Can you work these out from the model? Positions are in its coordinate system, mm. Coordinates: 2 decimals unless noted, no trailing zeros. Loops run counter-clockwise (first coordinate to the right, second up) from the corner with the lowest first, then second, coordinate; pieces in that order, holes last.
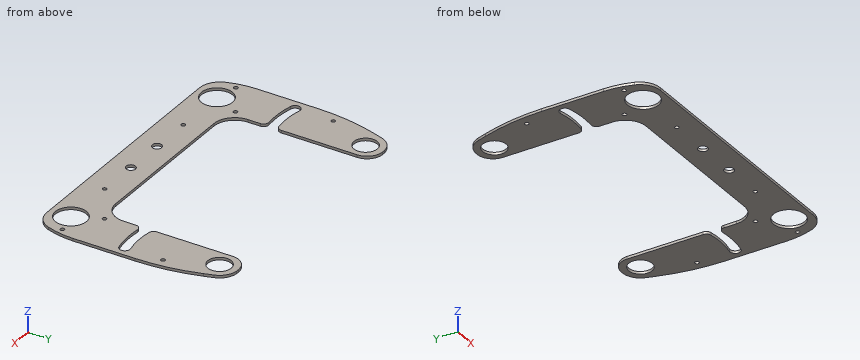
```python
from build123d import *

# Parameters (mm, degrees)
SKETCH1_R           = 14.2875
SKETCH1_R_2         = 19.05
SKETCH1_R_3         = 2.4892
SKETCH1_R_4         = 5.715
BOSS_EXTRUDE3_DEPTH = 3.175
SKETCH2_W           = 355.6
SKETCH2_H           = 19.05
CUT_EXTRUDE1_DEPTH  = 290.621961572
FILLET1_R           = 19.05
CUT_EXTRUDE2_DEPTH  = 290.621961572
FILLET2_R           = 254
CUT_EXTRUDE3_DEPTH  = 290.621961572
FILLET3_R           = 25.4
CUT_EXTRUDE4_DEPTH  = 290.621961572
FILLET4_R           = 6.35


with BuildPart() as part:
    # Sketch1 → Boss-Extrude3 (new body)
    with BuildSketch(Plane.XY):
        with BuildLine():
            Line((120.65, -152.4), (120.65, -6.35))
            Line((120.65, -6.35), (120.65, 6.35))
            ThreePointArc((120.65, 6.35), (124.369743879, 15.330256121), (133.35, 19.05))
            Line((133.35, 19.05), (165.1, 19.05))
            ThreePointArc((165.1, 19.05), (174.080256121, 15.330256121), (177.8, 6.35))
            Line((177.8, 6.35), (177.8, -6.35))
            Line((177.8, -6.35), (177.8, -222.25))
            ThreePointArc((177.8, -222.25), (175.940128061, -226.740128061), (171.45, -228.6))
            Line((171.45, -228.6), (12.7, -228.6))
            Line((12.7, -228.6), (-12.7, -228.6))
            Line((-12.7, -228.6), (-171.45, -228.6))
            ThreePointArc((-171.45, -228.6), (-175.940128061, -226.740128061), (-177.8, -222.25))
            Line((-177.8, -222.25), (-177.8, -6.35))
            Line((-177.8, -6.35), (-177.8, 6.35))
            ThreePointArc((-177.8, 6.35), (-174.080256121, 15.330256121), (-165.1, 19.05))
            Line((-165.1, 19.05), (-133.35, 19.05))
            ThreePointArc((-133.35, 19.05), (-124.369743879, 15.330256121), (-120.65, 6.35))
            Line((-120.65, 6.35), (-120.65, -6.35))
            Line((-120.65, -6.35), (-120.65, -152.4))
            ThreePointArc((-120.65, -152.4), (-113.210512242, -170.360512242), (-95.25, -177.8))
            Line((-95.25, -177.8), (-12.7, -177.8))
            Line((-12.7, -177.8), (12.7, -177.8))
            Line((12.7, -177.8), (95.25, -177.8))
            ThreePointArc((95.25, -177.8), (113.210512242, -170.360512242), (120.65, -152.4))
        make_face()
        with Locations((141.605, -22.02688)):
            Circle(SKETCH1_R, mode=Mode.SUBTRACT)
        with Locations(Location((-141.605, -22.02688, 0), (0, 0, 180))):
            Circle(SKETCH1_R, mode=Mode.SUBTRACT)
        with Locations((-141.605, -203.2)):
            Circle(SKETCH1_R_2, mode=Mode.SUBTRACT)
        with Locations(Location((141.605, -203.2, 0), (0, 0, 180))):
            Circle(SKETCH1_R_2, mode=Mode.SUBTRACT)
        with Locations((-76.2, -203.2)):
            Circle(SKETCH1_R_3, mode=Mode.SUBTRACT)
        with Locations(Location((76.2, -203.2, 0), (0, 0, 180))):
            Circle(SKETCH1_R_3, mode=Mode.SUBTRACT)
        with Locations((-25.4, -203.2)):
            Circle(SKETCH1_R_4, mode=Mode.SUBTRACT)
        with Locations((-149.225, 6.35)):
            Circle(SKETCH1_R_3, mode=Mode.SUBTRACT)
        with Locations(Location((149.225, 6.35, 0), (0, 0, 180))):
            Circle(SKETCH1_R_3, mode=Mode.SUBTRACT)
        with Locations((-168.275, -196.85)):
            Circle(SKETCH1_R_3, mode=Mode.SUBTRACT)
        with Locations(Location((168.275, -196.85, 0), (0, 0, 180))):
            Circle(SKETCH1_R_3, mode=Mode.SUBTRACT)
        with Locations((-165.1, -76.2)):
            Circle(SKETCH1_R_3, mode=Mode.SUBTRACT)
        with Locations(Location((165.1, -76.2, 0), (0, 0, 180))):
            Circle(SKETCH1_R_3, mode=Mode.SUBTRACT)
        with Locations((-127, -171.45)):
            Circle(SKETCH1_R_3, mode=Mode.SUBTRACT)
        with Locations(Location((127, -171.45, 0), (0, 0, 180))):
            Circle(SKETCH1_R_3, mode=Mode.SUBTRACT)
        with Locations(Location((25.4, -203.2, 0), (0, 0, 180))):
            Circle(SKETCH1_R_4, mode=Mode.SUBTRACT)
    extrude(amount=BOSS_EXTRUDE3_DEPTH)

    # Sketch2 → Cut-Extrude1 (cut, through all)
    with BuildSketch(Plane.XY.offset(3.175)):
        with Locations((0, 9.525)):
            Rectangle(SKETCH2_W, SKETCH2_H)
    extrude(amount=-CUT_EXTRUDE1_DEPTH, mode=Mode.SUBTRACT)

    # Fillet1
    fillet1_edges = [part.edges().sort_by_distance(p)[0] for p in [
        (-177.8, 0, 1.5875),
        (120.65, 0, 1.5875),
        (177.8, 0, 1.5875),
        (-120.65, 0, 1.5875),
    ]]
    fillet(fillet1_edges, radius=FILLET1_R)

    # Sketch3 → Cut-Extrude2 (cut, through all)
    with BuildSketch(Plane.XY.offset(3.175)):
        with BuildLine():
            Line((-177.8, 0), (-177.8, -63.5))
            Line((-177.8, -63.5), (-162.698792053, -15.403859213))
            ThreePointArc((-162.698792053, -15.403859213), (-155.445369527, -4.785747819), (-143.51, 0))
            Line((-143.51, 0), (-177.8, 0))
        make_face()
    cut_extrude2 = extrude(amount=-CUT_EXTRUDE2_DEPTH, mode=Mode.SUBTRACT)

    # Mirror1: Cut-Extrude2 across plane
    add(cut_extrude2.mirror(Plane.ZY), mode=Mode.SUBTRACT)

    # Fillet2
    fillet2_edges = [part.edges().sort_by_distance(p)[0] for p in [
        (-177.8, -63.5, 1.5875),
        (177.8, -63.5, 1.5875),
    ]]
    fillet(fillet2_edges, radius=FILLET2_R)

    # Sketch4 → Cut-Extrude3 (cut, through all)
    with BuildSketch(Plane.XY.offset(3.175)):
        with BuildLine():
            Line((-177.8, -177.8), (-177.8, -228.6))
            Line((-177.8, -228.6), (-164.188181024, -228.6))
            ThreePointArc((-164.188181024, -228.6), (-174.338063951, -204.096014982), (-177.8, -177.8))
        make_face()
        with BuildLine():
            Line((177.8, -177.8), (177.8, -228.6))
            Line((177.8, -228.6), (164.188181024, -228.6))
            ThreePointArc((164.188181024, -228.6), (174.338063951, -204.096014982), (177.8, -177.8))
        make_face()
    extrude(amount=-CUT_EXTRUDE3_DEPTH, mode=Mode.SUBTRACT)

    # Fillet3
    fillet3_edges = [part.edges().sort_by_distance(p)[0] for p in [
        (-164.188181024, -228.6, 1.5875),
        (164.188181024, -228.6, 1.5875),
    ]]
    fillet(fillet3_edges, radius=FILLET3_R)

    # Sketch5 → Cut-Extrude4 (cut, through all)
    with BuildSketch(Plane.XY.offset(3.175)):
        with BuildLine():
            Line((-120.65, -129.796193121), (-120.65, -116.826181287))
            ThreePointArc((-120.65, -116.826181287), (-142.167804376, -119.112938735), (-163.657650988, -116.576867488))
            ThreePointArc((-163.657650988, -116.576867488), (-171.284022099, -121.318540575), (-166.542349012, -128.944911687))
            ThreePointArc((-166.542349012, -128.944911687), (-143.641159604, -131.795686724), (-120.65, -129.796193121))
        make_face()
        with BuildLine():
            Line((120.65, -129.796193121), (120.65, -116.826181287))
            ThreePointArc((120.65, -116.826181287), (142.167804376, -119.112938735), (163.657650988, -116.576867488))
            ThreePointArc((163.657650988, -116.576867488), (171.284022099, -121.318540575), (166.542349012, -128.944911687))
            ThreePointArc((166.542349012, -128.944911687), (143.641159604, -131.795686724), (120.65, -129.796193121))
        make_face()
    extrude(amount=-CUT_EXTRUDE4_DEPTH, mode=Mode.SUBTRACT)

    # Fillet4
    fillet4_edges = [part.edges().sort_by_distance(p)[0] for p in [
        (-120.65, -116.826181287, 1.5875),
        (-120.65, -129.796193121, 1.5875),
        (120.65, -129.796193121, 1.5875),
        (120.65, -116.826181287, 1.5875),
    ]]
    fillet(fillet4_edges, radius=FILLET4_R)


solid = part.part
```
(1) I want a section at C-C on x = 86. Write out the boundary of the cut face in (y, z) (3 decimals), then the cut area to 3 significant figures.
Check values:
outline: (-228.6, 0) - (-177.8, 0) - (-177.8, 3.175) - (-228.6, 3.175) - close
area: 161 mm2
(2) I want a section at A-A on y = -107. Write out the boundary of the cut face in (x, z) (3 decimals).
Check values:
outline: (-177.8, 0) - (-120.65, 0) - (-120.65, 3.175) - (-177.8, 3.175) - close; (120.65, 0) - (177.8, 0) - (177.8, 3.175) - (120.65, 3.175) - close
(3) If I drill on probe 1 along Y at (x, z) = (-76.2, 2.25); probe 2 along X at (y, z) = (-75, 1.5); probe 3 along X at (y, z) = (-140, 2.95), over which ranges is the centre line in solid material (lowest first)?
Check values:
probe 1: y = -228.6 to -205.69, -200.71 to -177.8
probe 2: x = -176.31 to -167.28, -162.92 to -120.65, 120.65 to 162.92, 167.28 to 176.31
probe 3: x = -177.8 to -120.65, 120.65 to 177.8
(4) I want a section at B-B on x = -25.4. Write out the boundary of the cut face in (y, z) (3 decimals).
Check values:
outline: (-228.6, 0) - (-208.915, 0) - (-208.915, 3.175) - (-228.6, 3.175) - close; (-197.485, 0) - (-177.8, 0) - (-177.8, 3.175) - (-197.485, 3.175) - close
(5) I want a section at D-D on x = -101.5. Write out the boundary of the cut face in (y, z) (3 decimals).
Check values:
outline: (-228.6, 0) - (-177.019, 0) - (-177.019, 3.175) - (-228.6, 3.175) - close
(6) I'm going to push flat-ended pins straight in: pin 1 (1 mm diameter, centred on y = -59.5, z = 1, fed in from -X); pin 2 (1.6 mm diameter, centred on x = 2.5, z = 2.5, fed in from +Y); pin 3 (1.5 mm diameter, centred on y = -51, z = 1, fed in from -X). Where does each tip first touch, or does it pass through?
Check values:
pin 1: stops at x = -174.23
pin 2: stops at y = -177.8
pin 3: stops at x = -172.69
